Geometry: final body of the model. Coordinates: model frame, mm. Face numbers are marked on the shaded views. Coordinates: 2 decimals unless noted, no trailing zeros. Write each loop counter-clockwise with the first axis right and the second up, starting at its lowest first coordinate (ties: lowest second). Pieces come first, ordered by that corner, then holes. Notation, with made-up numbers: (41, 24.25) -> (66, 24.25) arc R20 cw to (66, 38.25) -> close; hole circle Ø9 at (0, 77). An arc over 180 degrees is marked (long way). One line per item, written item: value. Start each with the question number.
from build123d import *

# Parameters (mm, degrees)
F2_DEPTH = 40
F3_R     = 10
F4_R     = 10
F4_R_2   = 5
F5_DEPTH = 7.5


with BuildPart() as f2:
    # F1 (on Right) → F2 (new body)
    with BuildSketch(Plane.YZ):
        Polygon((175, 32.5), (175, 37.5), (-175, 37.5), (-175, 28.998962), (-170, 32.5), (170, 32.5), align=None)
        Polygon((282.111101, 37.5), (175, 37.5), (175, 32.5), (262.82962, 32.5), (175, -28.998962), (175, -37.5), align=None)
        Polygon((-175, 28.998962), (-175, 37.5), (-282.111101, -37.5), (-175, -37.5), (-175, -32.5), (-262.82962, -32.5), align=None)
        Polygon((175, -37.5), (175, -28.998962), (170, -32.5), (-170, -32.5), (-175, -32.5), (-175, -37.5), align=None)
    extrude(amount=F2_DEPTH)

    # F3
    f3_edges = [f2.edges().sort_by_distance(p)[0] for p in [
        (20, 282.111101, 37.5),
        (20, 262.82962, 32.5),
        (20, 170, -32.5),
        (20, -282.111101, -37.5),
        (20, -175, 37.5),
        (20, -170, 32.5),
        (20, -262.82962, -32.5),
        (20, 175, -37.5),
    ]]
    fillet(f3_edges, radius=F3_R)

    # F4 (on offset) → F5 (join, symmetric)
    with BuildSketch(Plane.YZ.offset(20)):
        with Locations((-166.847012, 22.5)):
            Circle(F4_R)
        with Locations((-166.847012, 22.5)):
            Circle(F4_R_2, mode=Mode.SUBTRACT)
        with Locations((-231.113672, -22.5)):
            Circle(F4_R)
        with Locations((-231.113672, -22.5)):
            Circle(F4_R_2, mode=Mode.SUBTRACT)
        with Locations((166.847012, -22.5)):
            Circle(F4_R)
        with Locations((166.847012, -22.5)):
            Circle(F4_R_2, mode=Mode.SUBTRACT)
        with Locations((231.113672, 22.5)):
            Circle(F4_R)
        with Locations((231.113672, 22.5)):
            Circle(F4_R_2, mode=Mode.SUBTRACT)
    extrude(amount=F5_DEPTH, both=True)


solid = f2.part
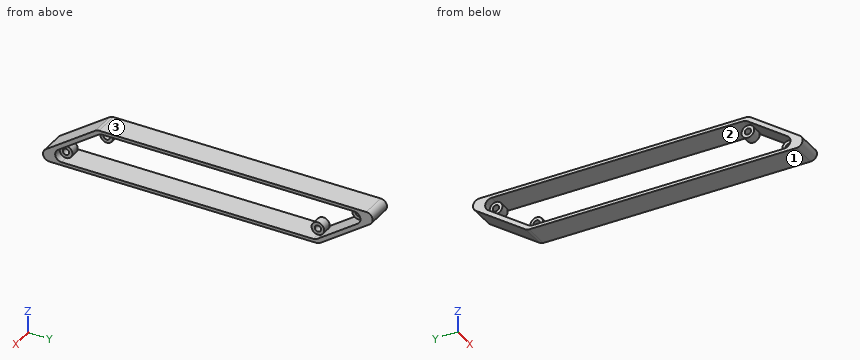
Q1. Draft query along Z for the marked faces 1, 2 and 3. Return one class per face: pulls with the +Z half, pulls with the -Z half, needs draft (parallel to the pull), parting line crosses it, or undercut.
Q2. First-contact query: P1, Ø6, axis at y = 166, z = -23.5, coming from the -X side; P2, Ø22, axis at y = -230, z = -18, coming from the -X side; P3, Ø10, axis at y = -230, z = -23, coming from the +X side; P4, Ø16, axis at y = 230.5, z = 23, coming from the -X side. Flat tips, straight axial feed; report the tip coordinate or a pass-through.
Q3. Cut plane A-A on x = 19. Output: boundary loops of the cut face in (y, z).
Q4. Cut plane B-B on y = 31. Output: boundary loops of the cut face in (x, z), and give its area (3 significant figures).
Q5. Cut plane C-C on z = 1. Output: boundary loops of the cut face in (x, y).
Q6. Line query: L1, parallel to Y at x = 21, z = 22; L2, parallel to Z at x = 32, y = 151; L3, parallel to X at y = 226, z = 26. Output: solid intervals per line, ascending. Write a range as from..to.
Solution:
1. face 1: pulls with the -Z half
1. face 2: undercut
1. face 3: pulls with the +Z half
2. P1: through
2. P2: x = 0
2. P3: x = 27.5
2. P4: x = 12.5
3. outline: (-256.13, -19.31) arc R10 ccw to (-250.4, -37.5) -> (171.85, -37.5) arc R10 ccw to (177.58, -35.69) -> (256.13, 19.31) arc R10 ccw to (250.4, 37.5) -> (-171.85, 37.5) arc R10 ccw to (-177.58, 35.69) -> close; hole (-236.85, -14.31) arc R10 cw (long way) to (-231.11, -32.5) -> (166.85, -32.5) arc R10 cw (long way) to (172.58, -30.69) -> (236.85, 14.31) arc R10 cw (long way) to (231.11, 32.5) -> (-166.85, 32.5) arc R10 cw (long way) to (-172.58, 30.69) -> close; hole circle Ø10 at (-231.11, -22.5); hole circle Ø10 at (-166.85, 22.5); hole circle Ø10 at (166.85, -22.5); hole circle Ø10 at (231.11, 22.5)
4. outline: (0, -37.5) -> (40, -37.5) -> (40, -32.5) -> (0, -32.5) -> close; (0, 32.5) -> (40, 32.5) -> (40, 37.5) -> (0, 37.5) -> close
4. area: 400 mm²
5. outline: (0, -227.13) -> (40, -227.13) -> (40, -214.99) -> (0, -214.99) -> close; (0, 217.84) -> (40, 217.84) -> (40, 229.98) -> (0, 229.98) -> close
6. L1: -197.14..-185, -176.83..-171.82, -161.87..-156.86, 221.13..226.14, 236.09..258.75
6. L2: -37.5..-32.5, 32.5..37.5
6. L3: 12.5..27.5
